Drawing for the job (mm, zero at the part's lowest x, y, z). A direction names the side the tool comes from. Round coordinates to 2 decimals unless told otherwise and drop trailing zeros. Write each loop counter-clockwise with the first axis right and the second up, starting at its lowest first coordinate (ties: lowest second). Pieces come first, ordered by that corner, then holes.
Item 1: Wall check: probe 1 along Y at (x, z) = (10, 2); probe 2 along X at (y, z) = (9, 5.5); probe 3 along X at (y, z) = (23.5, 2). Give the ranges that are in metal, low to high.
Item 2: Drop flat-ended pins along their axis: pin 1 Ø3.5 at (x, z) = (44.5, 5.5) entering from +Y; pin 2 Ø1.3 at (x, z) = (18.5, 5.5) entering from +Y; pin 3 Ø1.3 at (x, z) = (41.5, 3) entering from +Y. Give the stop position or say it passes through.
Item 3: Mould opens along X. For the marked faces 3, 4, 5 and 6 say: +X half, -X half, draft (parallel to the pull), parting line (faces both ways), or undercut.
Item 4: Band-saw the part on D-D, the plane x = 32. Write the cut outline in (y, z), then the cut area to 3 significant figures.
Item 5: Band-saw the part on A-A, the plane x = 10. Write the cut outline in (y, z), then the cut area to 3 significant figures.
Item 6: Band-saw the part on C-C, the plane z = 2.25. Write the cut outline in (x, y).
Item 7: 3-axis set-ups, long thin cutter, end or side, ignore diameter. For the marked faces 1 and 2: which of +Z, -Z, +X, -X, +Y, -Y reach the whole face in a straight line?
Item 8: Band-saw the part on B-B, the plane y = 8. Write the cut outline in (x, z), then the cut area to 3 significant figures.
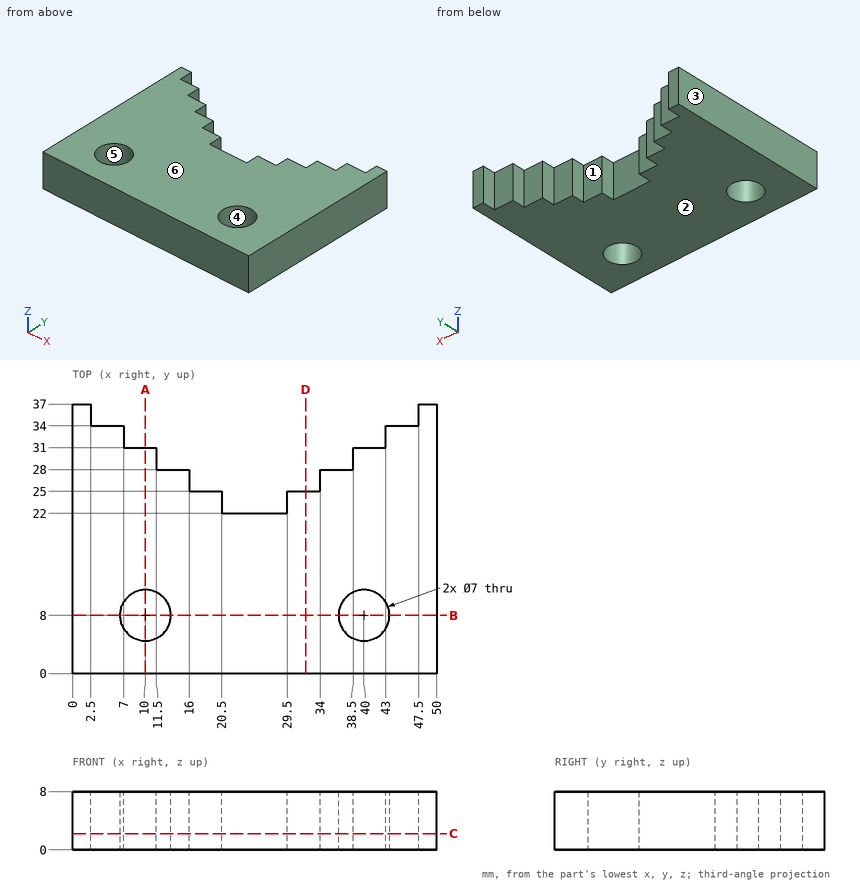
Results:
1. probe 1: y = 0 to 4.5, 11.5 to 31
1. probe 2: x = 0 to 6.65, 13.35 to 36.65, 43.35 to 50
1. probe 3: x = 0 to 20.5, 29.5 to 50
2. pin 1: stops at y = 34
2. pin 2: stops at y = 25
2. pin 3: stops at y = 31
3. face 3: -X half
3. face 4: undercut
3. face 5: undercut
3. face 6: draft
4. outline: (0, 0) - (25, 0) - (25, 8) - (0, 8) - close
4. area: 200 mm2
5. outline: (0, 0) - (4.5, 0) - (4.5, 8) - (0, 8) - close; (11.5, 0) - (31, 0) - (31, 8) - (11.5, 8) - close
5. area: 192 mm2
6. outline: (0, 0) - (50, 0) - (50, 37) - (47.5, 37) - (47.5, 34) - (43, 34) - (43, 31) - (38.5, 31) - (38.5, 28) - (34, 28) - (34, 25) - (29.5, 25) - (29.5, 22) - (20.5, 22) - (20.5, 25) - (16, 25) - (16, 28) - (11.5, 28) - (11.5, 31) - (7, 31) - (7, 34) - (2.5, 34) - (2.5, 37) - (0, 37) - close; hole circle Ø7 at (10, 8); hole circle Ø7 at (40, 8)
7. face 1: +Z, -Z, +Y
7. face 2: -Z, +X, -X, +Y, -Y
8. outline: (0, 0) - (6.5, 0) - (6.5, 8) - (0, 8) - close; (13.5, 0) - (36.5, 0) - (36.5, 8) - (13.5, 8) - close; (43.5, 0) - (50, 0) - (50, 8) - (43.5, 8) - close
8. area: 288 mm2
